Solid Edge part; units mm, degrees
sketch "Sketch1" plane through (0, 0, 0) normal (0, 0, 1) x (1, 0, 0)
  circle A0 centre (0, 0) radius 19.05
extrude "Protrusion1" add sketch "Sketch1" against normal blind 22.225
sketch "Sketch2" plane through (0, 0, 0) normal (0, 0, 1) x (1, 0, 0)
  line L0 (-22.225, -9.2059) -> (-9.2059, -22.225)
  line L1 (-9.2059, -22.225) -> (9.2059, -22.225)
  line L2 (9.2059, -22.225) -> (22.225, -9.2059)
  line L3 (22.225, -9.2059) -> (22.225, 9.2059)
  line L4 (22.225, 9.2059) -> (9.2059, 22.225)
  line L5 (9.2059, 22.225) -> (-9.2059, 22.225)
  line L6 (-9.2059, 22.225) -> (-22.225, 9.2059)
  line L7 (-22.225, 9.2059) -> (-22.225, -9.2059)
extrude "ExtrudedProtrusion_2" add sketch "Sketch2" along normal blind 12.7
chamfer "Chamfer_1" distance 3.1826 angle 45 8 edges at (15.7154, -15.7154, 12.7) (22.225, 0, 12.7) (15.7154, 15.7154, 12.7) (0, 22.225, 12.7) (-15.7154, 15.7154, 12.7) (-22.225, 0, 12.7) (-15.7154, -15.7154, 12.7) (0, -22.225, 12.7)
Input: part model. Units: mm. Frame: model coordinates. A direction names the side the tool comes from. Round coordinates to 2 decimals unless told otherwise and drop trailing zeros. Loops run counter-clockwise (first coordinate to the right, second up) from the corner with the lowest first, then second, coordinate; pieces in that order, holes last. Notation, with made-up numbers: M -34.5,69.25 L 4.5,69.25 A16 ccw 4.5,90.25 Z; hole C 74.25,-35 d3. An arc over 180 degrees is marked long. Answer as CSV lines item,"result". Start each with the question number.
(1) Reachability of faces 1 (the flat face through (18, 7, 0)), 2 (the flat face through (-14.48, -14.67, 11.13)) from +Z, -Z, +X, -X, +Y, -Y: full face, straight path, thin tool, end or side. Return the list, or none.
(2) First-contact query: pin 1 (1 mm diameter, centred on y = -3, z = -9, fed in from +X); pin 2 (12 mm diameter, centred on x = 10.5, z = -17, fed in from +Y); pin 3 (5 mm diameter, centred on x = 10, z = -14, fed in from +Y). Flat tips, straight axial feed; report the tip coordinate or a pass-through.
(3) Section B-B, the plane z = 2. Output: boundary loops of the cut face in (x, y) (3 decimals).
(4) Section A-A, the plane y = 0. Output: boundary loops of the cut face in (x, z) (3 decimals).
(5) Line query: line 1 (Y direction, x = 0, z = -17); line 2 (Z direction, x = -19, y = 4); line 3 (X direction, y = -0.5, z = -9). Output: solid intervals per line, ascending. Write a range as [from, to].
Values found:
1,face 1,"-Z"
1,face 2,"+Z, -X, -Y"
2,pin 1,"stops at x = 18.89"
2,pin 2,"stops at y = 18.51"
2,pin 3,"stops at y = 17.51"
3,outline,"M -22.225,-9.206 L -9.206,-22.225 L 9.206,-22.225 L 22.225,-9.206 L 22.225,9.206 L 9.206,22.225 L -9.206,22.225 L -22.225,9.206 Z"
4,outline,"M -22.225,0 L -19.05,0 L -19.05,-22.225 L 19.05,-22.225 L 19.05,0 L 22.225,0 L 22.225,9.517 L 19.042,12.7 L -19.042,12.7 L -22.225,9.517 Z"
5,line 1,"y = [-19.05, 19.05]"
5,line 2,"z = [0, 12.7]"
5,line 3,"x = [-19.04, 19.04]"
